Check sheet for the modelled part. Datum: model origin and axes. Units: mm. A direction names the side the tool comes from. Round coordinates to 2 decimals unless told otherwise and drop trailing zeros. Write each loop counter-clockwise with the first axis right and the second up, starting at its lowest first coordinate (ties: lowest second). Pieces come first, ordered by that corner, then holes. Notation, with made-up numbers: (-4.75, 25) - (27.25, 25) arc R26 ccw to (27.25, 56) - close; hole circle Ø2 at (37, 13). An arc over 180 degrees is marked (long way). Answer as a JSON object with one key per item and string values. Group by question number.
Item 1: Sectioned sample at D-D on z = -33.5. Record the boundary of the cut face in (x, y).
Item 2: Sectioned sample at C-C on x = -14. Record the boundary of the cut face in (y, z).
Item 3: Sectioned sample at B-B on x = -46. Record the boundary of the cut face in (y, z), plus the area to 3 significant figures.
Item 4: Thickness scan on line 1 (X direction, y = -2.25, z = -32.5); line 2 (X direction, y = -1.3, z = -51.5); line 3 (Z direction, x = -18.5, y = -3.65). Record the ranges inside material, lowest first.
Item 5: Sectioned sample at A-A on z = -24. Record the boundary of the cut face in (x, y), plus the area to 3 significant figures.
Item 6: Gauge pin test, flat ends, axial feed: P1, Ø6.5, axis at x = -54.69, z = -9.57, coming from the +Y side; P2, Ø3, axis at x = -48.5, y = -4, coming from the -Z side. Record the tip position at first contact, or that the pin passes through.
Item 7: Release check for a two-part mould opening along Z. For faces 3 (the flat face through (-50, -3, -63.377)), 4 (the flat face through (4.545, -3, -42)), 5 (the cylindrical face through (-20.93, -2.96, -7.51)), 6 (the cylindrical face through (-0.04, -2.96, -38.12)) record: pulls with the +Z half, pulls with the -Z half, needs draft (parallel to the pull), parting line crosses it, or undercut.
Item 8: Set-up check for faces 1 (the cylindrical face through (-52.73, -2.96, -18.52)), 2 (the flat face through (-39.553, -3, -73)): record each of +Z, -Z, +X, -X, +Y, -Y from which the full face is reachable in a straight line by a thin tool's end or side.
```python
from build123d import *

# Parameters (mm, degrees)
F0_R     = 2.25
F0_R_2   = 2.75
F0_R_3   = 2.2
F0_R_4   = 2.7
F0_R_5   = 12.3
F0_R_6   = 12.2
F0_R_7   = 2.15
F0_R_8   = 2.65
F0_R_9   = 2.1
F0_R_10  = 2.6
F0_R_11  = 2.05
F0_R_12  = 2.55
F0_R_13  = 2
F0_R_14  = 2.5
F0_R_15  = 12.1
F1_DEPTH = 6


with BuildPart() as f1:
    # F0 (on Front) → F1 (new body)
    with BuildSketch(Plane.XZ):
        Polygon((4.545036, 0), (0, 0), (-54.685275, 0), (-59.722289, 0), (-59.722289, -63.376926), (-39.553031, -63.376926), (-39.553031, -82.555786), (4.545036, -82.555786), align=None)
        with BuildLine():
            ThreePointArc((-28.561165, -74.508687), (-35.816369, -77.513891), (-32.811165, -70.258687))
            ThreePointArc((-32.811165, -70.258687), (-29.805961, -71.503483), (-28.561165, -74.508687))
        make_face(mode=Mode.SUBTRACT)
        with Locations((-54.685275, -57.419539)):
            Circle(F0_R, mode=Mode.SUBTRACT)
        with Locations((-45.115352, -57.419539)):
            Circle(F0_R_2, mode=Mode.SUBTRACT)
        with Locations((-54.685275, -47.849615)):
            Circle(F0_R_3, mode=Mode.SUBTRACT)
        with Locations((-45.115352, -47.849615)):
            Circle(F0_R_4, mode=Mode.SUBTRACT)
        with BuildLine():
            ThreePointArc((-32.811165, -65.720934), (-37.011165, -61.520934), (-32.811165, -57.320934))
            ThreePointArc((-32.811165, -57.320934), (-29.841316, -58.551086), (-28.611165, -61.520934))
            ThreePointArc((-28.611165, -61.520934), (-29.841316, -64.490783), (-32.811165, -65.720934))
        make_face(mode=Mode.SUBTRACT)
        with BuildLine():
            ThreePointArc((-32.811165, -52.683181), (-36.961165, -48.533181), (-32.811165, -44.383181))
            ThreePointArc((-32.811165, -44.383181), (-29.876672, -45.598688), (-28.661165, -48.533181))
            ThreePointArc((-28.661165, -48.533181), (-29.876672, -51.467675), (-32.811165, -52.683181))
        make_face(mode=Mode.SUBTRACT)
        with Locations((-11.215762, -67.734145)):
            Circle(F0_R_5, mode=Mode.SUBTRACT)
        with Locations((-11.673733, -41.788895)):
            Circle(F0_R_6, mode=Mode.SUBTRACT)
        with Locations((-54.685275, -38.279692)):
            Circle(F0_R_7, mode=Mode.SUBTRACT)
        with Locations((-45.115352, -38.279692)):
            Circle(F0_R_8, mode=Mode.SUBTRACT)
        with Locations((-54.685275, -28.709769)):
            Circle(F0_R_9, mode=Mode.SUBTRACT)
        with Locations((-45.115352, -28.709769)):
            Circle(F0_R_10, mode=Mode.SUBTRACT)
        with BuildLine():
            ThreePointArc((-32.811165, -39.645429), (-36.911165, -35.545429), (-32.811165, -31.445429))
            ThreePointArc((-32.811165, -31.445429), (-29.912027, -32.646291), (-28.711165, -35.545429))
            ThreePointArc((-28.711165, -35.545429), (-29.912027, -38.444566), (-32.811165, -39.645429))
        make_face(mode=Mode.SUBTRACT)
        with BuildLine():
            ThreePointArc((-32.811165, -26.607676), (-36.861165, -22.557676), (-32.811165, -18.507676))
            ThreePointArc((-32.811165, -18.507676), (-29.947382, -19.693893), (-28.761165, -22.557676))
            ThreePointArc((-28.761165, -22.557676), (-29.947382, -25.421458), (-32.811165, -26.607676))
        make_face(mode=Mode.SUBTRACT)
        with Locations((-54.685275, -19.139846)):
            Circle(F0_R_11, mode=Mode.SUBTRACT)
        with Locations((-45.115352, -19.139846)):
            Circle(F0_R_12, mode=Mode.SUBTRACT)
        with Locations((-54.685275, -9.569923)):
            Circle(F0_R_13, mode=Mode.SUBTRACT)
        with Locations((-45.115352, -9.569923)):
            Circle(F0_R_14, mode=Mode.SUBTRACT)
        with BuildLine():
            ThreePointArc((-32.811165, -13.569923), (-35.639592, -6.741496), (-28.811165, -9.569923))
            ThreePointArc((-28.811165, -9.569923), (-29.982738, -12.39835), (-32.811165, -13.569923))
        make_face(mode=Mode.SUBTRACT)
        with Locations((-12.010878, -15.684631)):
            Circle(F0_R_15, mode=Mode.SUBTRACT)
    extrude(amount=F1_DEPTH)


solid = f1.part
```
Completed:
{
 "1": {"outline": "(-59.72, -6) - (-36.36, -6) - (-36.36, 0) - (-59.72, 0) - close; (-29.26, -6) - (-20.63, -6) - (-20.63, 0) - (-29.26, 0) - close; (-2.72, -6) - (4.55, -6) - (4.55, 0) - (-2.72, 0) - close"},
 "2": {"outline": "(-6, -82.56) - (0, -82.56) - (0, -79.71) - (-6, -79.71) - close; (-6, -55.75) - (0, -55.75) - (0, -53.77) - (-6, -53.77) - close; (-6, -29.81) - (0, -29.81) - (0, -27.62) - (-6, -27.62) - close; (-6, -3.75) - (0, -3.75) - (0, 0) - (-6, 0) - close"},
 "3": {"outline": "(-6, -63.38) - (0, -63.38) - (0, -60.02) - (-6, -60.02) - close; (-6, -54.82) - (0, -54.82) - (0, -50.4) - (-6, -50.4) - close; (-6, -45.3) - (0, -45.3) - (0, -40.78) - (-6, -40.78) - close; (-6, -35.78) - (0, -35.78) - (0, -31.15) - (-6, -31.15) - close; (-6, -26.26) - (0, -26.26) - (0, -21.53) - (-6, -21.53) - close; (-6, -16.75) - (0, -16.75) - (0, -11.91) - (-6, -11.91) - close; (-6, -7.23) - (0, -7.23) - (0, 0) - (-6, 0) - close", "area": "202 mm²"},
 "4": {"line 1": "-59.72 to -35.56, -30.07 to -19.58, -3.76 to 4.55", "line 2": "-59.72 to -35.71, -29.91 to -19.06, -4.29 to 4.55", "line 3": "-82.56 to -77.65, -57.82 to -51.9, -31.68 to -25.9, -5.47 to 0"},
 "5": {"outline": "(-59.72, -6) - (-36.6, -6) - (-36.6, 0) - (-59.72, 0) - close; (-29.03, -6) - (-20.8, -6) - (-20.8, 0) - (-29.03, 0) - close; (-3.22, -6) - (4.55, -6) - (4.55, 0) - (-3.22, 0) - close", "area": "235 mm²"},
 "6": {"P1": "y = 0", "P2": "z = -63.38"},
 "7": {"face 3": "pulls with the -Z half", "face 4": "needs draft", "face 5": "undercut", "face 6": "undercut"},
 "8": {"face 1": "+Y, -Y", "face 2": "-Z, -X, +Y, -Y"}
}
